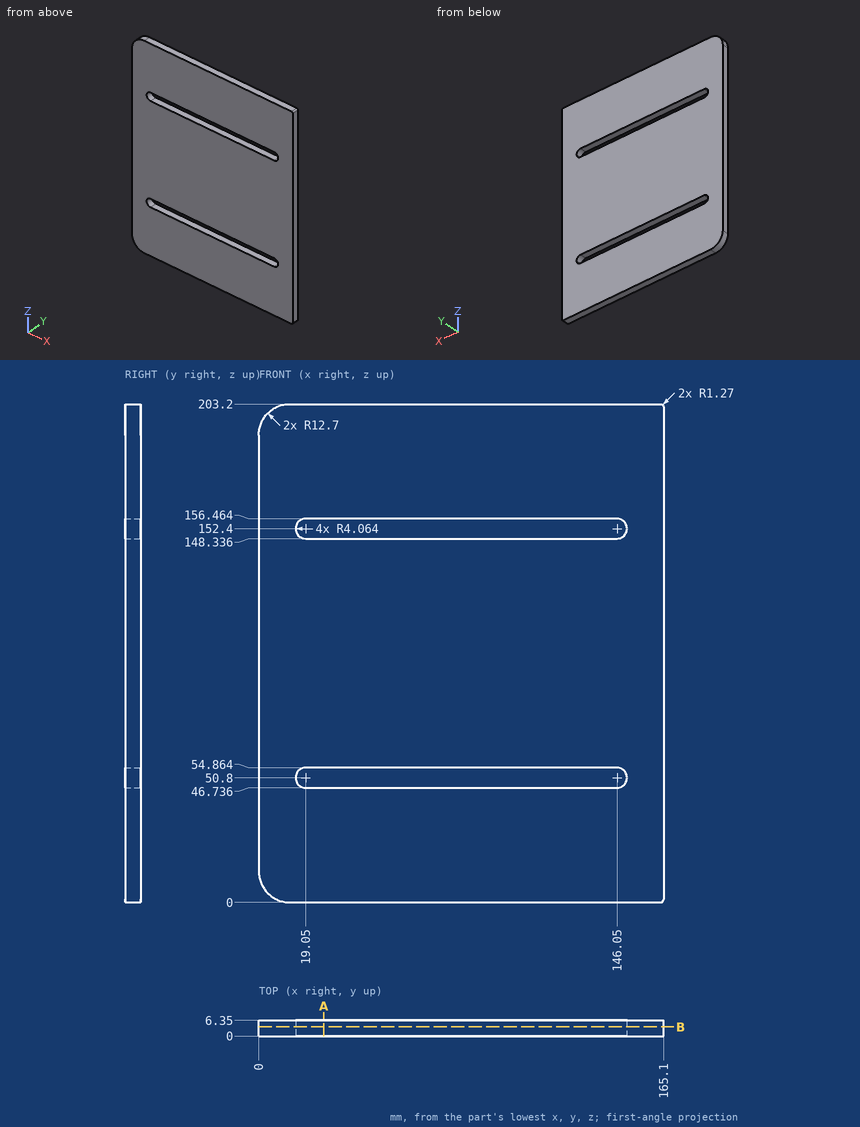
For this review, use the dimensioned drawing (mm, ordinates from the lowest corner) and the shaded views. Coordinates: 2 decimals unless noted, no trailing zeros. Loops run counter-clockwise (first coordinate to the right, second up) from the corner with the lowest first, then second, coordinate; pieces in that order, holes last. Notation, with made-up numbers: (5.25, 17) -> (33.25, 17) arc R22 cw to (33.25, 53) -> close; hole circle Ø1 at (-35, 67.25). An arc over 180 degrees is marked (long way). Return JSON: item names as keys, results as strings. Group by question number.
(1) Consider section B-B, the plane y = 3.75. Give the boundary of the cut face in (x, z).
(2) Consider section A-A, the plane x = 26.5. Give the boundary of the cut face in (y, z), plus the area to 3 significant figures.
(3) To check wall thickness, follow L1, parallel to Z at x = 132, y = 3.75; L2, parallel to X at y = 3.75, z = 152.5; L3, parallel to X at y = 0.5, z = 193. State the ranges of each line that lie inside material, in increasing order.
Results below:
{
 "1": {"outline": "(0, 12.7) arc R12.7 ccw to (12.7, 0) -> (163.83, 0) arc R1.27 ccw to (165.1, 1.27) -> (165.1, 201.93) arc R1.27 ccw to (163.83, 203.2) -> (12.7, 203.2) arc R12.7 ccw to (0, 190.5) -> close; hole (19.05, 46.74) -> (146.05, 46.74) arc R4.06 ccw to (146.05, 54.86) -> (19.05, 54.86) arc R4.06 ccw to start; hole (19.05, 148.34) -> (146.05, 148.34) arc R4.06 ccw to (146.05, 156.46) -> (19.05, 156.46) arc R4.06 ccw to start"},
 "2": {"outline": "(0, 0) -> (6.35, 0) -> (6.35, 46.74) -> (0, 46.74) -> close; (0, 54.86) -> (6.35, 54.86) -> (6.35, 148.34) -> (0, 148.34) -> close; (0, 156.46) -> (6.35, 156.46) -> (6.35, 203.2) -> (0, 203.2) -> close", "area": "1,190 mm2"},
 "3": {"L1": "z = 0 to 46.74, 54.86 to 148.34, 156.46 to 203.2", "L2": "x = 0 to 14.99, 150.11 to 165.1", "L3": "x = 0.25 to 165.1"}
}
